```python
from build123d import *

# Parameters (mm, degrees)
F0_W     = 281.793315
F0_H     = 50.8
F1_DEPTH = 3.81
F2_W     = 25.273
F2_H     = 3.048
F3_DEPTH = 25.4
F5_DEPTH = 25.4


with BuildPart() as f1:
    # F0 (on Front) → F1 (new body)
    with BuildSketch(Plane.XZ):
        with Locations((18.189594, -20.427606)):
            Rectangle(F0_W, F0_H)
    extrude(amount=F1_DEPTH)

    # F2 (on face) → F3 (cut)
    with BuildSketch(Plane.XZ.offset(3.81)):
        with Locations((70.503751, -1.390693)):
            Rectangle(F2_W, F2_H)
        with Locations((70.503751, -39.464519)):
            Rectangle(F2_W, F2_H)
        with Locations((-76.110764, -1.390693)):
            Rectangle(F2_W, F2_H)
        with Locations((-76.110764, -39.464519)):
            Rectangle(F2_W, F2_H)
    extrude(amount=-F3_DEPTH, mode=Mode.SUBTRACT)

    # F4 (on face) → F5 (cut)
    with BuildSketch(Plane.XZ.offset(3.81)):
        Polygon((111.503996, -15.1832), (67.158138, -15.1832), (57.92642, -15.1832), (57.92642, -26.221192), (67.158138, -26.221192), (111.503996, -26.221192), align=None)
    extrude(amount=-F5_DEPTH, mode=Mode.SUBTRACT)


solid = f1.part
```
The listing builds one solid part. Answer for the finished solid, in the listing's coordinates (mm). Coordinates: 2 decimals unless noted, no trailing zeros. Write each loop counter-clockwise with the first axis right and the second up, starting at its lowest first coordinate (ties: lowest second). Pieces come first, ordered by that corner, then holes. Notation, with made-up numbers: (-28, 58) - (-11, 58) arc R18 cw to (-11, 68) - close; hole circle Ø1 at (-6, 75). An arc over 180 degrees is marked (long way). One line per item, written item: value.
1) Find section C-C (y = -1.5). Give the vertices of the cut face in (x, z), and give its area (3 significant figures).
Geometry check:
outline: (-122.71, -45.83) - (159.09, -45.83) - (159.09, 4.97) - (-122.71, 4.97) - close; hole (-88.75, -40.99) - (-63.47, -40.99) - (-63.47, -37.94) - (-88.75, -37.94) - close; hole (-88.75, -2.91) - (-63.47, -2.91) - (-63.47, 0.13) - (-88.75, 0.13) - close; hole (57.87, -40.99) - (83.14, -40.99) - (83.14, -37.94) - (57.87, -37.94) - close; hole (57.87, -2.91) - (83.14, -2.91) - (83.14, 0.13) - (57.87, 0.13) - close; hole (57.93, -26.22) - (111.5, -26.22) - (111.5, -15.18) - (57.93, -15.18) - close
area: 13,400 mm2
2) Consider line 1 along Z through (x, y) = (61.5, -0.4); line 2 along X through (y, z) = (-0.2, -1); line 3 along X through (y, z) = (-1.1, -21.5). Determine where each line is inside the solid, lowest interval first. Write a range as from..to.
Geometry check:
line 1: z = -45.83..-40.99, -37.94..-26.22, -15.18..-2.91, 0.13..4.97
line 2: x = -122.71..-88.75, -63.47..57.87, 83.14..159.09
line 3: x = -122.71..57.93, 111.5..159.09
3) Find section A-A (z = -19). Give the vertices of the cut face in (x, y).
Geometry check:
outline: (-122.71, -3.81) - (57.93, -3.81) - (57.93, 0) - (-122.71, 0) - close; (111.5, -3.81) - (159.09, -3.81) - (159.09, 0) - (111.5, 0) - close
4) Find section B-B (x = 100). Give the vertices of the cut face in (y, z).
Geometry check:
outline: (-3.81, -45.83) - (0, -45.83) - (0, -26.22) - (-3.81, -26.22) - close; (-3.81, -15.18) - (0, -15.18) - (0, 4.97) - (-3.81, 4.97) - close
5) Find section D-D (x = 61.5). Give the vertices of the cut face in (y, z).
Geometry check:
outline: (-3.81, -45.83) - (0, -45.83) - (0, -40.99) - (-3.81, -40.99) - close; (-3.81, -37.94) - (0, -37.94) - (0, -26.22) - (-3.81, -26.22) - close; (-3.81, -15.18) - (0, -15.18) - (0, -2.91) - (-3.81, -2.91) - close; (-3.81, 0.13) - (0, 0.13) - (0, 4.97) - (-3.81, 4.97) - close
